Job drawing, mm, ordinate dimensions from the low corner. One solid piece. A direction names the side the tool comes from. Give positions to 0.01 mm unless a question says otherwise; leave off trailing zeros. Order: outer loops, then holes, each group sorted by start corner. A loop starts at its lowest first (then second) coordinate and runs counter-clockwise, first axis right, second up. Notation, with made-up numbers: (24, 22.25) - (66, 22.25) arc R21 ccw to (66, 35.25) - close; hole circle Ø1 at (-33, 64). An arc over 180 degrees is marked (long way). One line per item, written item: value.
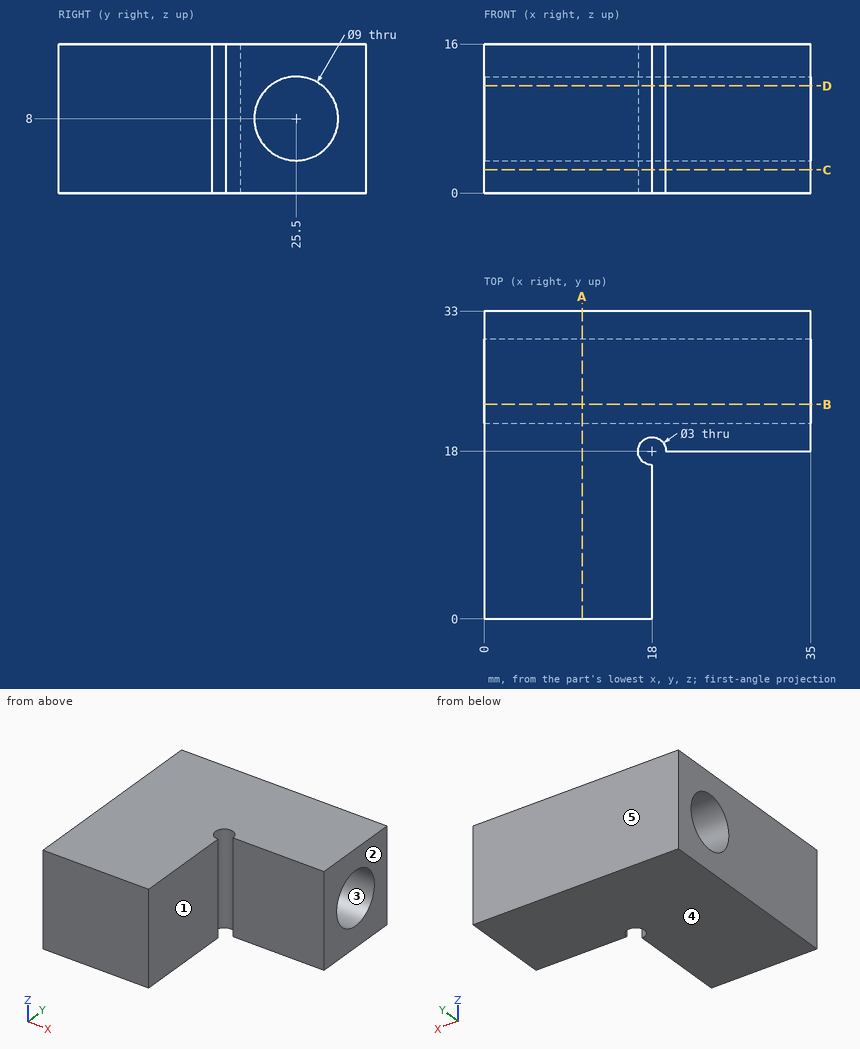
1) Slice it at B-B on y = 23. Write the cut outline in (x, z), then the cut area to 3 significant figures.
Answer:
outline: (0, 0) - (35, 0) - (35, 4.26) - (0, 4.26) - close; (0, 11.74) - (35, 11.74) - (35, 16) - (0, 16) - close
area: 298 mm2
2) Which spindle directions (+Z, -Z, +X, -X, +Y, -Y) get a long thin tool onto all of the face, cutting with end or side? Do the marked faces 1 and 2. Say none if no direction does.
Answer:
face 1: +Z, -Z, +X, -Y
face 2: +Z, -Z, +X, +Y, -Y
3) Slice it at C-C on z = 2.5. Write the cut outline in (x, y).
Answer:
outline: (0, 0) - (18, 0) - (18, 16.5) arc R1.5 cw (long way) to (19.5, 18) - (35, 18) - (35, 33) - (0, 33) - close
4) Drop flat-ended pins along their axis: P1, Ø8, axis at x = 26.5, z = 9, coming from the -Y side; P2, Ø5, axis at y = 10, z = 11, coming from the +X side. Give the stop position or say it passes through.
Answer:
P1: stops at y = 18
P2: stops at x = 18
5) Wall check: line 1 along Z through (x, y) = (13, 25.5); line 2 along X through (y, z) = (5.5, 10.5); line 3 along Y through (x, z) = (4, 9.5). Give the ranges that are in metal, low to high. Write a range as [from, to].
Answer:
line 1: z = [0, 3.5], [12.5, 16]
line 2: x = [0, 18]
line 3: y = [0, 21.26], [29.74, 33]
6) Slice it at D-D on z = 11.5. Write the cut outline in (x, y).
Answer:
outline: (0, 0) - (18, 0) - (18, 16.5) arc R1.5 cw (long way) to (19.5, 18) - (35, 18) - (35, 22.67) - (0, 22.67) - close; (0, 28.33) - (35, 28.33) - (35, 33) - (0, 33) - close
7) Two-plate mould, pull along Z, no slides. Class the marked faces 3, 4 and 5: pulls with the +Z half, pulls with the -Z half, needs draft (parallel to the pull), parting line crosses it, or undercut.
Answer:
face 3: undercut
face 4: pulls with the -Z half
face 5: needs draft
8) Slice it at A-A on x = 10.5. Write the cut outline in (y, z), then the cut area to 3 significant figures.
Answer:
outline: (0, 0) - (33, 0) - (33, 16) - (0, 16) - close; hole circle Ø9 at (25.5, 8)
area: 464 mm2
